The drawing under review shows one solid part. Ordinate dimensions are in mm from its lowest x, y, z. A direction names the side the tool comes from. Coordinates: 2 decimals unless noted, no trailing zeros. Write each loop counter-clockwise with the first axis right and the second up, starting at its lowest first coordinate (ties: lowest second). Pieces come first, ordered by that corner, then holes. Notation, with made-up numbers: (-35.5, -37.75) - (-9.5, -37.75) arc R20 ccw to (-9.5, -2.75) - close; hole circle Ø11 at (35, -33.75). An arc over 180 degrees is marked (long way). Answer as CSV lines item,"result". Start each with the question number.
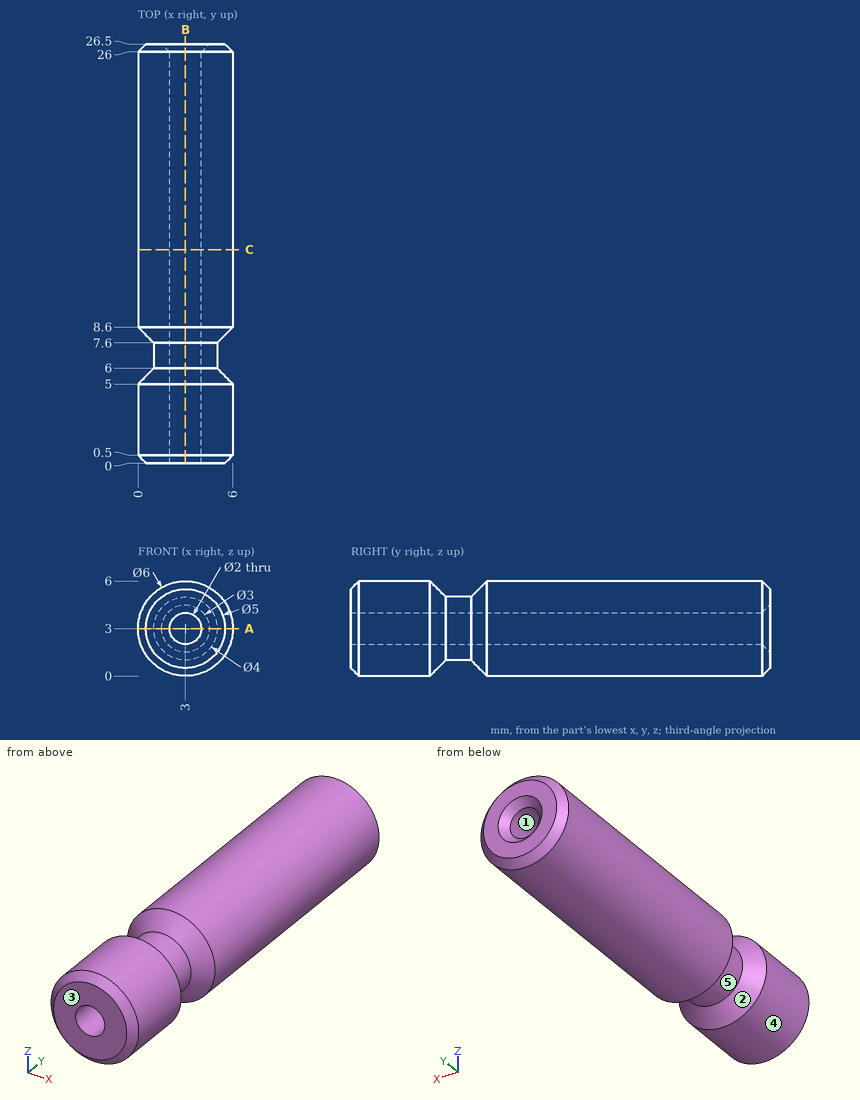
(1) Add section A-A on z = 3. Give the boundary of the cut face in (x, y), then the cut area to 3 significant figures.
(2) The part is to be moulded in two halves that separate along Z. For the marked faces 1, 2 and 3, say which applies: released by +Z, released by -Z, zero draft, split by the parting line, or undercut.
(3) For the marked faces 4 and 5, list the 3-axis set-ups (+Z, -Z, +X, -X, +Y, -Y) from which the entire face can be reached by the end or side of a thin tool; tool diameter is ignored.
(4) Add section B-B on x = 3. Give the boundary of the cut face in (y, z), then the cut area to 3 significant figures.
(5) Wall thickness on line 1 (Z direction, x = 3, y = 16.25); line 2 (Z direction, x = 3, y = 5.5); line 3 (Y direction, x = 2.05, z = 5.1): over which ranges is each line inside the solid? List them lowest first.
(6) Add section C-C on y = 13.5. Give the boundary of the cut face in (x, z).
Reported:
1,outline,"(0, 0.5) - (0.5, 0) - (2, 0) - (2, 26) - (1.5, 26.5) - (0.5, 26.5) - (0, 26) - (0, 8.6) - (1, 7.6) - (1, 6) - (0, 5) - close; (4, 0) - (5.5, 0) - (6, 0.5) - (6, 5) - (5, 6) - (5, 7.6) - (6, 8.6) - (6, 26) - (5.5, 26.5) - (4.5, 26.5) - (4, 26) - close"
1,area,"100 mm²"
2,face 1,"undercut"
2,face 2,"split by the parting line"
2,face 3,"zero draft"
3,face 4,"+Y, -Y"
3,face 5,"none"
4,outline,"(0, 0.5) - (0.5, 0) - (5, 0) - (6, 1) - (7.6, 1) - (8.6, 0) - (26, 0) - (26.5, 0.5) - (26.5, 1.5) - (26, 2) - (0, 2) - close; (0, 4) - (26, 4) - (26.5, 4.5) - (26.5, 5.5) - (26, 6) - (8.6, 6) - (7.6, 5) - (6, 5) - (5, 6) - (0.5, 6) - (0, 5.5) - close"
4,area,"100 mm²"
5,line 1,"0 to 2, 4 to 6"
5,line 2,"0.5 to 2, 4 to 5.5"
5,line 3,"0 to 5.7, 7.9 to 26.5"
6,outline,"circle Ø6 at (3, 3); hole circle Ø2 at (3, 3)"
